Could you check a few things on this model? Use its own coordinates, in mm. Coordinates: 2 decimals unless noted, no trailing zeros. Loops run counter-clockwise (first coordinate to the right, second up) from the corner with the lowest first, then second, coordinate; pieces in that order, holes last.
from build123d import *

# Parameters (mm, degrees)
SKETCH1_R             = 3.81
SKETCH1_R_2           = 3.41
BOSS_EXTRUDE1_DEPTH   = 0.325
SKETCH1_R_3           = 2.8
BOSS_EXTRUDE1_2_DEPTH = 0.325
SKETCH1_3_R           = 3.41
SKETCH1_3_R_2         = 2.8
BOSS_EXTRUDE2_DEPTH   = 0.24


with BuildPart() as part:
    # Sketch1 → Boss-Extrude1 (new body)
    with BuildSketch(Plane(origin=(0, 0, 0), x_dir=(1, 0, 0), z_dir=(0, 1, 0))):
        with Locations(Location((0, 0, 0), (0, 0, 270))):
            Circle(SKETCH1_R)
        with Locations(Location((0, 0, 0), (0, 0, 270))):
            Circle(SKETCH1_R_2, mode=Mode.SUBTRACT)
    extrude(amount=BOSS_EXTRUDE1_DEPTH)



with BuildPart() as body_2:
    # Sketch1 → Boss-Extrude1 2 (new body)
    with BuildSketch(Plane(origin=(0, 0, 0), x_dir=(1, 0, 0), z_dir=(0, 1, 0))):
        with Locations(Location((0, 0, 0), (0, 0, 270))):
            Circle(SKETCH1_R_3)
    extrude(amount=BOSS_EXTRUDE1_2_DEPTH)


with BuildPart() as part_1:
    add(part.part)

    add(body_2.part)  # Boss-Extrude2 merges body 2
    # Sketch1_3 → Boss-Extrude2 (add)
    # profile 1 of 2: a face of its own
    with BuildSketch(Plane(origin=(0, 0, 0), x_dir=(1, 0, 0), z_dir=(0, 1, 0))):
        with BuildLine():
            Line((-3.175, -2.106056742), (-3.175, -34.29))
            Line((-3.175, -34.29), (3.175, -34.29))
            Line((3.175, -34.29), (3.175, -2.106056742))
            ThreePointArc((3.175, -2.106056742), (0, -3.81), (-3.175, -2.106056742))
        make_face()
    # profile 2 of 2: a face of its own
    with BuildSketch(Plane(origin=(0, 0, 0), x_dir=(1, 0, 0), z_dir=(0, 1, 0))):
        Circle(SKETCH1_3_R)
        Circle(SKETCH1_3_R_2, mode=Mode.SUBTRACT)
    extrude(amount=BOSS_EXTRUDE2_DEPTH)


solid = part_1.part
(1) Imagine slicing it at A-A, the plane z = 0. Write out the boundary of the cut face in (x, y) (3 decimals), and give its area (3 significant figures).
Answers:
outline: (-3.81, 0) - (3.81, 0) - (3.81, 0.325) - (3.41, 0.325) - (3.41, 0.24) - (2.8, 0.24) - (2.8, 0.325) - (-2.8, 0.325) - (-2.8, 0.24) - (-3.41, 0.24) - (-3.41, 0.325) - (-3.81, 0.325) - close
area: 2.37 mm2
(2) For pin 1 (3 mm diameter, centred on x = 0, z = 18.5, fed in from +Y), with a flat end and sliding along its axis, tell me the tip position at first contact or that it passes through.
Answers:
pin 1: stops at y = 0.24
(3) I need wall thicknesses on probe 1 along Y at (x, z) = (-1.5, 17.5); probe 2 along X at (y, z) = (0.15, 28) (3 decimals); probe 3 along Z at (x, y) = (3.25, 0.15). Which ranges of each line are inside material? Lowest first, please.
Answers:
probe 1: y = 0 to 0.24
probe 2: x = -3.175 to 3.175
probe 3: z = -1.99 to 1.99
(4) Imagine slicing it at C-C, the plane y = 0.05. Write out the boundary of the cut face in (x, z) (3 decimals), and give its area (3 significant figures).
Answers:
outline: (-3.175, 2.106) arc R3.81 ccw (long way) to (3.175, 2.106) - (3.175, 34.29) - (-3.175, 34.29) - close
area: 242 mm2
(5) Imagine slicing it at B-B, the plane x = 0. Write out the boundary of the cut face in (y, z) (3 decimals).
Answers:
outline: (0, -3.81) - (0.325, -3.81) - (0.325, -3.41) - (0.24, -3.41) - (0.24, -2.8) - (0.325, -2.8) - (0.325, 2.8) - (0.24, 2.8) - (0.24, 3.41) - (0.325, 3.41) - (0.325, 3.81) - (0.24, 3.81) - (0.24, 34.29) - (0, 34.29) - close
(6) We'd pull the mould along Z, two halves only. Please class faces 1 (the face through (-2, 0.325, -3)), 2 (the face through (0.168, 0.16, -3.806)), 3 (the face through (0, 0.24, -3)): +Z half, -Z half, draft (parallel to the pull), parting line (faces both ways), or undercut.
Answers:
face 1: draft
face 2: parting line
face 3: undercut
(7) Imagine slicing it at D-D, the plane x = -1.5. Write out the boundary of the cut face in (y, z) (3 decimals).
Answers:
outline: (0, -3.502) - (0.325, -3.502) - (0.325, -3.062) - (0.24, -3.062) - (0.24, -2.364) - (0.325, -2.364) - (0.325, 2.364) - (0.24, 2.364) - (0.24, 3.062) - (0.325, 3.062) - (0.325, 3.502) - (0.24, 3.502) - (0.24, 34.29) - (0, 34.29) - close
